Autodesk Inventor part; units mm, degrees
ref_plane "YZ Plane" through (0, 0, 0) normal (1, 0, 0) x (0, 1, 0)
ref_plane "XZ Plane" through (0, 0, 0) normal (0, 1, 0) x (-1, 0, 0)
ref_plane "XY Plane" through (0, 0, 0) normal (0, 0, 1) x (1, 0, 0)
sketch "Sketch1" plane through (0, 0, 0) normal (0, 1, 0) x (-1, 0, 0)
  line L0 (0, 0) -> (-19.5, 0)
  line L1 (-19.5, 0) -> (-19.5, -134)
  line L2 (-19.5, -134) -> (0, -134)
  line L3 (0, -134) -> (0, 0)
  line L4 (2, 2) -> (-21.5, 2)
  line L5 (-21.5, 2) -> (-21.5, -136)
  line L6 (-21.5, -136) -> (2, -136)
  line L7 (2, -136) -> (2, 2)
  line L8 (-2.5, -22) -> (-16.5, -22)
  line L9 (-16.5, -22) -> (-16.5, -131.25)
  line L10 (-16.5, -131.25) -> (-2.5, -131.25)
  line L11 (-2.5, -131.25) -> (-2.5, -22)
  line L12 (-2.5, -22) -> (0, -22)
  line L13 (-2.5, -22) -> (0, -22) construction
  line L14 (-16.5, -22) -> (-19.5, -22)
  line L15 (-16.5, -22) -> (-13.5, -22) construction
  line L16 (-6.724, -131.25) -> (-3.974, -131.25) construction
  line L17 (-6, -131.25) -> (-6, -134)
  line L18 (-2.5, -128) -> (0, -128)
  line L19 (-3.25, 2) -> (-16.25, 2)
  line L20 (-16.25, 2) -> (-16.25, 0)
  line L21 (-16.25, 0) -> (-3.25, 0)
  line L22 (-3.25, 0) -> (-3.25, 2)
  line L23 (-19.5, 0) -> (-21.5, 0)
  line L24 (-21.5, 0) -> (-21.5, 2)
  line L25 (-21.5, 2) -> (-19.5, 2)
  line L26 (-19.5, 2) -> (-19.5, 0)
  line L27 (0, 0) -> (2, 0)
  line L28 (2, 0) -> (2, 2)
  line L29 (2, 2) -> (0, 2)
  line L30 (0, 2) -> (0, 0)
  line L31 (0, -134) -> (2, -134)
  line L32 (2, -134) -> (2, -136)
  line L33 (2, -136) -> (0, -136)
  line L34 (0, -136) -> (0, -134)
  line L35 (-19.5, -134) -> (-21.5, -134)
  line L36 (-21.5, -134) -> (-21.5, -136)
  line L37 (-21.5, -136) -> (-19.5, -136)
  line L38 (-19.5, -136) -> (-19.5, -134)
  dimension "d0" = 19.5
  dimension "d1" = 134
  dimension "d2" = 2
  dimension "d3" = 2
  dimension "d4" = 2
  dimension "d5" = 2
  dimension "d6" = 14
  dimension "d7" = 109.25
  dimension "d8" = 22
  dimension "d9" = 2.5
  dimension "d10" = 0
  dimension "d11" = 180
  dimension "d17" = 6
  dimension "d18" = 6
  dimension "d20" = 13
  dimension "d21" = 5.25
extrude "Extrusion1" add sketch "Sketch1" against normal blind 11
extrude "Extrusion2" cut sketch "Sketch1" against normal blind 10 contours L3 L12 L8 L14 L1 L0 | L3 L2 L17 L10 L11 L18 | L11 L10 L9 L8
fillet "Fillet1" radius 1 4 edges at (2.5, -5, -128) (1.25, 0, -128) (6, 0, -132.625) (6, -5, -131.25)
extrude "Extrusion3" cut sketch "Sketch1" against normal blind 7 contours L0 L20 L4 L22
extrude "Extrusion5" add sketch "Sketch1" along normal blind 2 contours L27 L7 L31 L3 | L34 L6 L38 L2
sketch "Sketch2" plane through (0, 0, 0) normal (0, 1, 0) x (1, 0, 0)
  line L0 (19.5, 0) -> (0, 0)
  line L1 (19.5, 0) -> (21.5, 0)
  line L2 (21.5, 0) -> (21.5, 134)
  line L3 (21.5, 134) -> (19.5, 134)
  line L4 (19.5, 134) -> (19.5, 0)
  line L5 (16.25, -2) -> (3.25, -2)
  line L6 (19.5, 0) -> (16.25, 0)
  line L7 (16.25, 0) -> (16.25, -2)
  line L8 (16.25, -2) -> (19.5, -2)
  line L9 (19.5, -2) -> (19.5, 0)
  line L10 (-2, -2) -> (3.25, -2)
  line L11 (0, 0) -> (3.25, 0)
  line L12 (3.25, 0) -> (3.25, -2)
  line L13 (3.25, -2) -> (0, -2)
  line L14 (0, -2) -> (0, 0)
  dimension "d28" = 2
  dimension "d29" = 134
extrude "Extrusion6" add sketch "Sketch2" along normal blind 2 contours L9 L8 L7 L0 | L4 L3 L2 L1 | L12 L10 L14 L0
properties part number "case-bottom"
Could you check a few things on this model? Use its own coordinates, in mm. A direction names the side the tool comes from. Give positions to 0.01 mm unless a question says otherwise; leave off trailing zeros. Order: outer loops, then holes, each group sorted by start corner. A loop starts at its lowest first (then second) coordinate and runs counter-clockwise, first axis right, second up. Notation, with made-up numbers: (24, 44.25) - (79, 44.25) arc R16 cw to (79, 59.25) - close; hole circle Ø10 at (70.5, 77). An arc over 180 degrees is marked (long way). Return JSON: item names as keys, results as strings. Group by question number.
Q1. Will these pins go through, and if not, where does the flat tip stop? pin 1 Ø3 at (x, z) = (8, -93) entering from +Y; pin 2 Ø1 at (x, y) = (11, -0.5) entering from +Z; pin 3 Ø0.6 at (y, z) = (1.5, 1) entering from +X; pin 4 Ø1.6 at (x, z) = (-1, -134.5) entering from +Y.
Q2. Please list where these lines run through material, in increasing order: line 1 along X through (y, z) = (-3.5, -68.5); line 2 along X through (y, z) = (0.75, -97); line 3 along Z through (x, y) = (17.5, -4.5). Write a range as [from, to].
Q3. Suppose I cut it at D-D, the plane z = -7. Please give me the cut outline in (x, y), and give its area (3 significant figures).
Q4. Suppose I cut it at B-B, the plane z = -109.5. Please give me the cut outline in (x, y), and give its area (4 significant figures).
Q5. Suppose I cut it at C-C, the plane y = -3.75. Please give me the cut outline in (x, z), and give its area (3 significant figures).
Q6. Which directions (+Z, -Z, +X, -X, +Y, -Y) give clear straight access to the entire face, cutting with the end or side of a thin tool? Please do faces 4 (the face through (10, -4, -136)), 5 (the face through (7, -8, 0)).
Q7. Thinking about a two-plate mould opening in X: for faces 1 (the face through (17, 0, -82)), 2 (the face through (9.6, -7.3, 2)), 3 (the face through (-2, -4, -68)), which applies, pulls with the +X half, pulls with the -X half, needs draft (parallel to the pull), parting line crosses it, or undercut?
Q8. Suppose I cut it at A-A, the plane x = 9.75. Please give me the cut outline in (y, z).
Resolved:
{
 "1": {"pin 1": "stops at y = -10", "pin 2": "stops at z = -131.25", "pin 3": "stops at x = 19.5", "pin 4": "stops at y = 2"},
 "2": {"line 1": "x = [-2, 2.5], [16.5, 21.5]", "line 2": "x = [-2, 0], [19.5, 21.5]", "line 3": "z = [-136, -22], [0, 2]"},
 "3": {"outline": "(-2, -11) - (21.5, -11) - (21.5, 2) - (19.5, 2) - (19.5, -10) - (0, -10) - (0, 2) - (-2, 2) - close", "area": "71.5 mm2"},
 "4": {"outline": "(-2, -11) - (21.5, -11) - (21.5, 2) - (19.5, 2) - (19.5, 0) - (16.5, 0) - (16.5, -10) - (2.5, -10) - (2.5, 0) - (0, 0) - (0, 2) - (-2, 2) - close", "area": "126.5 mm2"},
 "5": {"outline": "(-2, -136) - (21.5, -136) - (21.5, 2) - (16.25, 2) - (16.25, 0) - (19.5, 0) - (19.5, -22) - (16.5, -22) - (16.5, -131.25) - (7, -131.25) arc R1 ccw to (6, -132.25) - (6, -134) - (0, -134) - (0, -128) - (1.5, -128) arc R1 ccw to (2.5, -127) - (2.5, -22) - (0, -22) - (0, 0) - (3.25, 0) - (3.25, 2) - (-2, 2) - close", "area": "1,230 mm2"},
 "6": {"face 4": "-Z, +X, -X, +Y, -Y", "face 5": "+Y"},
 "7": {"face 1": "undercut", "face 2": "needs draft", "face 3": "pulls with the -X half"},
 "8": {"outline": "(-11, -136) - (2, -136) - (2, -134) - (0, -134) - (0, -131.25) - (-10, -131.25) - (-10, 0) - (-7, 0) - (-7, 2) - (-11, 2) - close"}
}
